Input: part model. Units: mm. Frame: model coordinates. A direction names the side the tool comes from. Round coordinates to 2 decimals unless told otherwise and drop trailing zeros. Loops run counter-clockwise (first coordinate to the right, second up) from the corner with the lowest first, then second, coordinate; pieces in that order, holes last. Notation, with made-up numbers: (4, -33) - (22, -33) arc R19 ccw to (22, 0) - close; hole circle Ø7 at (-7, -33). An arc over 180 degrees is marked (long way). Write each question's results on one line, items separated by ' | '.
from build123d import *

# Parameters (mm, degrees)
F0_W      = 11.5
F0_H      = 6
F1_DEPTH  = 15
F2_W      = 11.3
F2_H      = 11.3
F3_DEPTH  = 24
F5_W      = 12.6701932168
F5_H      = 0.4
F6_DEPTH  = 5.2
F7_W      = 9.9
F7_H      = 0.3
F8_DEPTH  = 6
F9_D      = 4.9
F10_DEPTH = 3.5


with BuildPart() as f1:
    # F0 (on Front) → F1 (new body)
    with BuildSketch(Plane.XZ):
        with BuildLine():
            ThreePointArc((11.5, 6), (5.75, 11.75), (0, 6))
            Line((0, 6), (11.5, 6))
        make_face()
        with Locations((5.75, 3)):
            Rectangle(F0_W, F0_H)
    extrude(amount=F1_DEPTH)

    # F2 (on face) → F3 (join)
    with BuildSketch(Plane.XZ.offset(15)):
        with Locations((5.75, 5.65)):
            Rectangle(F2_W, F2_H)
    extrude(amount=F3_DEPTH)

    # F5 (on 3pt) → F6 (cut)
    with BuildSketch(Plane(origin=(0, 0, 6), x_dir=(1, 0, 0), z_dir=(0, 0, -1))):
        with Locations((6.4887672779, 12.7)):
            Rectangle(F5_W, F5_H)
    extrude(amount=-F6_DEPTH, mode=Mode.SUBTRACT)

    # F7 (on face) → F8 (cut, through all)
    with BuildSketch(Plane(origin=(0, 0, 0), x_dir=(1, 0, 0), z_dir=(0, 0, -1))):
        with Locations((5.75, 12.7)):
            Rectangle(F7_W, F7_H)
    extrude(amount=-F8_DEPTH, mode=Mode.SUBTRACT)

    # F9 (through all)
    with Locations(Plane(origin=(0, 0, 0), x_dir=(1, 0, 0), z_dir=(0, 0, -1))):
        with Locations((5.65, 29)):
            Hole(F9_D / 2)

    # F5 (on 3pt) → F10 (cut)
    with BuildSketch(Plane(origin=(0, 0, 6), x_dir=(1, 0, 0), z_dir=(0, 0, -1))):
        with Locations((6.4887672779, 12.7)):
            Rectangle(F5_W, F5_H)
    extrude(amount=F10_DEPTH, mode=Mode.SUBTRACT)


solid = f1.part
1. Section query A-A, the plane y = -29. Output: boundary loops of the cut face in (x, z).
Answer:
outline: (0.1, 0) - (3.2, 0) - (3.2, 11.3) - (0.1, 11.3) - close; (8.1, 0) - (11.4, 0) - (11.4, 11.3) - (8.1, 11.3) - close
2. Contact query for flat-ended pins moving along their axis: pin 1 (1.5 mm diameter, centred on y = -14.5, z = 8, fed in from +X); pin 2 (5.5 mm diameter, centred on x = 5.65, y = -29, fed in from +Z); pin 3 (1 mm diameter, centred on x = 3.5, y = -11.5, fed in from +Z); pin 4 (2.5 mm diameter, centred on x = 9, z = 8, fed in from +Y). Output: stop coordinate, or through.
Answer:
pin 1: x = 11.4 | pin 2: z = 11.3 | pin 3: z = 11.48 | pin 4: y = 0
3. Line query: line 1 (Y direction, x = 5.65, z = 3.5); line 2 (X direction, y = -29, z = 8.25); line 3 (Y direction, x = 10, z = 8.75). Output: solid intervals per line, ascending. Write a range as [from, to].
Answer:
line 1: [-39, -31.45], [-26.55, -12.9], [-12.5, 0] | line 2: [0.1, 3.2], [8.1, 11.4] | line 3: [-39, -12.9], [-12.5, 0]
4. Section query D-D, the plane y = -8. Output: boundary loops of the cut face in (x, z), plus the area to 3 significant figures.
Answer:
outline: (0, 0) - (11.5, 0) - (11.5, 6) arc R5.75 ccw to (0, 6) - close | area: 121 mm^2
5. Set-up query: faces 4 (the flat face through (6, -12.9, 7)), 5 (the cylindrical face through (5.88, -7.4, 11.75)), 6 (the flat face through (3, -27, 11.3)), 7 (the flat face through (11.4, -27, 6)), 8 (the flat face through (0.1, -27, 6)). Return all of +Z, -Z, +X, -X, +Y, -Y with unobstructed straight access to the full face (end or side cutting, diameter ignored); none if empty.
Answer:
face 4: +X | face 5: +Z, +Y | face 6: +Z, +X, -X, -Y | face 7: +Z, -Z, +X, -Y | face 8: +Z, -Z, -X, -Y
6. Section query B-B, the plane x = 5.75. Output: boundary loops of the cut face in (y, z).
Answer:
outline: (-39, 0) - (-31.45, 0) - (-31.45, 11.3) - (-39, 11.3) - close; (-26.55, 0) - (-12.85, 0) - (-12.85, 2.5) - (-12.9, 2.5) - (-12.9, 11.2) - (-12.5, 11.2) - (-12.5, 2.5) - (-12.55, 2.5) - (-12.55, 0) - (0, 0) - (0, 11.75) - (-15, 11.75) - (-15, 11.3) - (-26.55, 11.3) - close
7. Section query C-C, the plane z = 6.5. Output: boundary loops of the cut face in (x, y).
Answer:
outline: (0.02, -15) - (0.1, -15) - (0.1, -39) - (11.4, -39) - (11.4, -15) - (11.48, -15) - (11.48, -12.9) - (0.15, -12.9) - (0.15, -12.5) - (11.48, -12.5) - (11.48, 0) - (0.02, 0) - close; hole circle Ø4.9 at (5.65, -29)
8. Mould query, pull axis X, two halves, no side actions, for faces 1 (the flat face through (6, -39, 6)), 2 (the flat face through (6, -12.85, 1)), 3 (the flat face through (0, -7, 3)). Classes: pulls with the +X half, pulls with the -X half, needs draft (parallel to the pull), parting line crosses it, or undercut.
Answer:
face 1: needs draft | face 2: undercut | face 3: pulls with the -X half
